from build123d import *

# Parameters (mm, degrees)
SKETCH1_R           = 1.75
BOSS_EXTRUDE1_DEPTH = 3
CUT_EXTRUDE1_DEPTH  = 1


with BuildPart() as part:
    # Sketch1 → Boss-Extrude1 (new body)
    with BuildSketch(Plane(origin=(0, 0, 0), x_dir=(1, 0, 0), z_dir=(0, 1, 0))):
        with BuildLine():
            Line((23.900635095, -8.602885683), (19.823061771, -6.248697627))
            ThreePointArc((19.823061771, -6.248697627), (18.239104498, -4.560898425), (17.855232358, -2.278305828))
            ThreePointArc((17.855232358, -2.278305828), (15.588457268, 9), (6.954545455, 16.602237726))
            ThreePointArc((6.954545455, 16.602237726), (5.169698348, 18.07597705), (4.5, 20.291623888))
            Line((4.5, 20.291623888), (4.5, 25))
            ThreePointArc((4.5, 25), (0, 29.5), (-4.5, 25))
            Line((-4.5, 25), (-4.5, 21.073284825))
            ThreePointArc((-4.5, 21.073284825), (-2.892304845, 15.073284825), (1.5, 10.68097998))
            Line((1.5, 10.68097998), (5, 8.660254038))
            ThreePointArc((5, 8.660254038), (8.660254038, -5), (-5, -8.660254038))
            Line((-5, -8.660254038), (-8.5, -6.639528096))
            ThreePointArc((-8.5, -6.639528096), (-14.5, -5.031832941), (-20.5, -6.639528096))
            Line((-20.5, -6.639528096), (-23.900635095, -8.602885683))
            ThreePointArc((-23.900635095, -8.602885683), (-25.547749412, -14.75), (-19.400635095, -16.397114317))
            Line((-19.400635095, -16.397114317), (-15.323061771, -14.042926261))
            ThreePointArc((-15.323061771, -14.042926261), (-13.069406149, -13.515078625), (-10.900686903, -14.323931899))
            ThreePointArc((-10.900686903, -14.323931899), (0, -18), (10.900686903, -14.323931899))
            ThreePointArc((10.900686903, -14.323931899), (13.069406149, -13.515078625), (15.323061771, -14.042926261))
            Line((15.323061771, -14.042926261), (19.400635095, -16.397114317))
            ThreePointArc((19.400635095, -16.397114317), (25.547749412, -14.75), (23.900635095, -8.602885683))
        make_face()
        with Locations((0, 25)):
            Circle(SKETCH1_R, mode=Mode.SUBTRACT)
        with Locations((21.650635095, -12.5)):
            Circle(SKETCH1_R, mode=Mode.SUBTRACT)
        with Locations((-21.650635095, -12.5)):
            Circle(SKETCH1_R, mode=Mode.SUBTRACT)
    extrude(amount=BOSS_EXTRUDE1_DEPTH)

    # Sketch2 → Cut-Extrude1 (cut)
    with BuildSketch(Plane(origin=(0, 3, 0), x_dir=(1, 0, 0), z_dir=(0, 1, 0))):
        Polygon((2.8, 23.383419246), (2.8, 26.616580754), (0, 28.233161507), (-2.8, 26.616580754), (-2.8, 23.383419246), (0, 21.766838493), align=None)
        Polygon((24.450635095, -14.116580754), (24.450635095, -10.883419246), (21.650635095, -9.266838493), (18.850635095, -10.883419246), (18.850635095, -14.116580754), (21.650635095, -15.733161507), align=None)
        Polygon((-24.450635095, -14.116580754), (-21.650635095, -15.733161507), (-18.850635095, -14.116580754), (-18.850635095, -10.883419246), (-21.650635095, -9.266838493), (-24.450635095, -10.883419246), align=None)
    extrude(amount=-CUT_EXTRUDE1_DEPTH, mode=Mode.SUBTRACT)


solid = part.part
For this review, take the finished solid that the model builds, in its own axes (mm). A direction names the side the tool comes from. Round coordinates to 2 decimals unless told otherwise and drop trailing zeros. Order: outer loops, then holes, each group sorted by start corner. A loop starts at its lowest first (then second) coordinate and runs counter-clockwise, first axis right, second up. Notation, with made-up numbers: (19.25, -37) -> (46.25, -37) arc R32 cw to (46.25, -10) -> close; hole circle Ø4 at (73.5, -34.5). An arc over 180 degrees is marked (long way). Write item = value, one per line. Start each with the question number.
1) Insertion check: pin 1 (1 mm diameter, centred on x = 2.5, y = 0.5, fed in from -Z); pin 2 (0.5 mm diameter, centred on y = 2.5, z = 13, fed in from -X); pin 3 (0.5 mm diameter, centred on y = 2.5, z = 13, fed in from +X). Each pin has a flat end and moves straight along its axis. Give the tip position at first contact, or say it passes through.
2) To check wall thickness, follow line 1 (X direction, y = 2.45, z = -25); line 2 (X direction, y = 0.95, z = 12); line 3 (X direction, y = 0.5, z = -25). State the ranges of each line that lie inside material, in increasing order. Write a range as from..to.
3) Take a section at D-D on z = 0. State the section outline as (x, y) points, plus the area to 3 significant figures.
4) Take a section at B-B on x = 3.5. State the section outline as (y, z) points.
5) Take a section at A-A on z = 12.5. State the section outline as (x, y) points.
6) Take a section at C-C on y = 0.45. State the section outline as (x, z) points.
7) Tool access review of faces 5 (the face through (-14.412, 1.479, 5.032)), 6 (the face through (23.07, 2.507, 10.086)), 7 (the face through (-4.5, 1, -23)): name each direction out of +Z, -Z, +X, -X, +Y, -Y from which nothing blocks a thin tool from reaching the whole face with its end or side.
8) The part is to be moulded in two halves that separate along Z. For faces 1 (the face through (0.1, 1.5, -29.5)), 2 (the face through (3.2, 1.5, -9.7)), 3 (the face through (10, 0, 3)), 4 (the face through (-17.39, 1.479, 15.236)), say which applies: +Z half, -Z half, draft (parallel to the pull), parting line (faces both ways), or undercut.
Verdict:
q1.pin_1 = -29.03
q1.pin_2 = -26.14
q1.pin_3 = 26.14
q2.line_1 = -4.5..-2.8, 2.8..4.5
q2.line_2 = -26.12..-23.33, -19.97..19.97, 23.33..26.12
q2.line_3 = -4.5..-1.75, 1.75..4.5
q3.outline = (10, 0) -> (18, 0) -> (18, 3) -> (10, 3) -> close
q3.area = 24.0 mm2
q4.outline = (0, -27.83) -> (3, -27.83) -> (3, -9.53) -> (0, -9.53) -> close; (0, 9.37) -> (3, 9.37) -> (3, 17.66) -> (0, 17.66) -> close
q5.outline = (-26.15, 0) -> (-23.4, 0) -> (-23.4, 2) -> (-24.45, 2) -> (-24.45, 3) -> (-26.15, 3) -> close; (-19.9, 0) -> (19.9, 0) -> (19.9, 2) -> (18.85, 2) -> (18.85, 3) -> (-18.85, 3) -> (-18.85, 2) -> (-19.9, 2) -> close; (23.4, 0) -> (26.15, 0) -> (26.15, 3) -> (24.45, 3) -> (24.45, 2) -> (23.4, 2) -> close
q6.outline = (-23.9, 8.6) -> (-20.5, 6.64) arc R12 ccw to (-8.5, 6.64) -> (-5, 8.66) arc R10 cw to (5, -8.66) -> (1.5, -10.68) arc R12 ccw to (-4.5, -21.07) -> (-4.5, -25) arc R4.5 ccw to (4.5, -25) -> (4.5, -20.29) arc R4 cw to (6.95, -16.6) arc R18 ccw to (17.86, 2.28) arc R4 cw to (19.82, 6.25) -> (23.9, 8.6) arc R4.5 ccw to (19.4, 16.4) -> (15.32, 14.04) arc R4 cw to (10.9, 14.32) arc R18 ccw to (-10.9, 14.32) arc R4 cw to (-15.32, 14.04) -> (-19.4, 16.4) arc R4.5 ccw to start; hole circle Ø3.5 at (-21.65, 12.5); hole circle Ø3.5 at (0, -25); hole circle Ø3.5 at (21.65, 12.5)
q7.face_5 = -Z, +Y, -Y
q7.face_6 = +Y
q7.face_7 = -Z, -X, +Y, -Y
q8.face_1 = -Z half
q8.face_2 = undercut
q8.face_3 = draft
q8.face_4 = +Z half
